For this review, take the finished solid that the model builds, in its own axes (mm). A direction names the side the tool comes from. Give positions to 0.01 mm unless a question says otherwise; leave off trailing zeros. Loops run counter-clockwise (first coordinate to the right, second up) from the corner with the lowest first, then second, coordinate; pieces in that order, holes last. Notation, with made-up numbers: (67.5, 31) - (83.5, 31) arc R15 cw to (83.5, 38) - close; hole circle Ø3 at (14, -9). An arc over 180 degrees is marked (long way). Put each result on its own line as item: value.
from build123d import *

# Parameters (mm, degrees)
BASPROSKE_W         = 44.5
BASPROSKE_H         = 30
TOOTHCUT_DEPTH      = 62.483737687
TEETHCUTS_COUNT     = 22
TEETHCUTS_ANGLE     = 343.636363636
HUBNEAONESKE_R      = 21
HUBNEARONE_DEPTH    = 5.5000508
BORSKE_R            = 12
BORE_DEPTH          = 50.0000508
CUT_EXTRUDE1_START  = -15.41
SKETCH1_R           = 30
CUT_EXTRUDE1_DEPTH  = 15.41
BOSS_EXTRUDE1_START = -3.95
SKETCH2_R           = 12
BOSS_EXTRUDE1_DEPTH = 3.95
SKETCH3_R           = 1.26
CUT_EXTRUDE2_DEPTH  = 55.622234789
SKETCH4_R           = 17.7
CUT_EXTRUDE3_DEPTH  = 30.64


with BuildPart() as part:
    # BasProSke → Base-Revolve (revolve)
    with BuildSketch(Plane(origin=(0, 0, 0), x_dir=(1, 0, 0), z_dir=(0, 1, 0)), mode=Mode.PRIVATE) as base_revolve_sk:
        with Locations((22.25, 15)):
            Rectangle(BASPROSKE_W, BASPROSKE_H)
    revolve(base_revolve_sk.sketch.rotate(Axis((-10, 0, 0), (1, 0, 0)), 180), axis=Axis((-10, 0, 0), (1, 0, 0)))

    # TooCutSke → ToothCut (cut, through all)
    with BuildSketch(Plane(origin=(0, 0, 0), x_dir=(0, 0, -1), z_dir=(1, 0, 0))):
        with BuildLine():
            ThreePointArc((1.215293185, 24.343683749), (0, 24.374), (-1.215293185, 24.343683749))
            ThreePointArc((-1.215293185, 24.343683749), (-2.034367134, 27.241050063), (-3.608361155, 29.807790507))
            ThreePointArc((-3.608361155, 29.807790507), (0, 30.0254), (3.608361155, 29.807790507))
            ThreePointArc((3.608361155, 29.807790507), (2.034367134, 27.241050063), (1.215293185, 24.343683749))
        make_face()
    toothcut = extrude(amount=TOOTHCUT_DEPTH, mode=Mode.SUBTRACT)

    # TeethCuts: ToothCut ×22 about axis
    teethcuts_axis = Axis((-10, 0, 0), (1, 0, 0))
    for i in range(1, TEETHCUTS_COUNT):
        add(toothcut.rotate(teethcuts_axis, i * TEETHCUTS_ANGLE / (TEETHCUTS_COUNT - 1)), mode=Mode.SUBTRACT)

    # HubNeaOneSke → HubNearOne (add)
    with BuildSketch(Plane.ZY):
        with Locations(Location((0, 0, 0), (0, 0, 180))):
            Circle(HUBNEAONESKE_R)
    extrude(amount=HUBNEARONE_DEPTH)

    # BorSke → Bore (cut, symmetric)
    with BuildSketch(Plane(origin=(0, 0, 0), x_dir=(0, 0, -1), z_dir=(1, 0, 0))):
        with Locations(Location((0, 0, 0), (0, 0, 180))):
            Circle(BORSKE_R)
    extrude(amount=BORE_DEPTH, both=True, mode=Mode.SUBTRACT)

    # Sketch1 → Cut-Extrude1 (cut)
    with BuildSketch(Plane.ZY.offset(5.5000508).offset(CUT_EXTRUDE1_START)):
        Circle(SKETCH1_R)
    extrude(amount=CUT_EXTRUDE1_DEPTH, mode=Mode.SUBTRACT)

    # Sketch2 → Boss-Extrude1 (add)
    with BuildSketch(Plane.ZY.offset(-9.9099492).offset(BOSS_EXTRUDE1_START)):
        Circle(SKETCH2_R)
    extrude(amount=BOSS_EXTRUDE1_DEPTH)

    # Sketch3 → Cut-Extrude2 (cut, through all)
    with BuildSketch(Plane.ZY.offset(-9.9099492)):
        with Locations((0, 8)):
            Circle(SKETCH3_R)
        with Locations((6.92820323, 4)):
            Circle(SKETCH3_R)
        with Locations((6.92820323, -4)):
            Circle(SKETCH3_R)
        with Locations((0, -8)):
            Circle(SKETCH3_R)
        with Locations((-6.92820323, -4)):
            Circle(SKETCH3_R)
        with Locations((-6.92820323, 4)):
            Circle(SKETCH3_R)
    extrude(amount=-CUT_EXTRUDE2_DEPTH, mode=Mode.SUBTRACT)

    # Sketch4 → Cut-Extrude3 (cut)
    with BuildSketch(Plane(origin=(44.5, 0, 0), x_dir=(0, 0, -1), z_dir=(1, 0, 0))):
        Circle(SKETCH4_R)
    extrude(amount=-CUT_EXTRUDE3_DEPTH, mode=Mode.SUBTRACT)


solid = part.part
1) For faces 5 (the face through (26.963, -13.187, -23.952)), 6 (the face through (26.96, -26.74, -5.72)), 7 (the face through (26.963, -21.785, -16.392)), list the 3-axis set-ups (+Z, -Z, +X, -X, +Y, -Y) from which the entire face can be reached by the end or side of a thin tool; tool diameter is ignored.
Geometry check:
face 5: -Z, +X, -X
face 6: +X, -X
face 7: +X, -X, -Y
2) Take a section at A-A on z = 0. State how many separate pieces and enclosed holes the cut face has, and give its area (3 significant figures).
Geometry check:
separate pieces: 3
enclosed holes: 0
area: 582 mm²
3) Insertion check: pin 1 Ø1 at (x, z) = (21.5, -24) entering from +Y; pin 2 Ø1.5 at (y, z) = (-8, 0) entering from +X (3 decimals); pin 3 Ø3 at (x, y) = (39.5, -2) entering from +Z; pin 4 Ø1.5 at (y, z) = (5.5, -5.5) entering from +X. Each pin has a flat end and moves straight along its axis. Give the tip position at first contact, or say it passes through.
Geometry check:
pin 1: stops at y = 16.78
pin 2: passes through
pin 3: stops at z = 30
pin 4: stops at x = 13.86
4) Wall thickness on line 1 (Y direction, x = 35, z = -26); line 2 (Y direction, x = 16, z = -22.5); line 3 (Y direction, x = 22, z = 9): over which ranges is each line inside the solid? List them lowest first.
Geometry check:
line 1: y = -9.47 to -5.5, -2.13 to 2.13, 5.5 to 9.47
line 2: y = -16.46 to -11.83, -9.37 to 9.37, 11.83 to 16.46
line 3: y = -24.74 to -15.24, 15.24 to 24.74
5) Take a section at B-B on y = 13.5. State the section outline as (x, z) points.
Geometry check:
outline: (9.91, -24.22) - (44.5, -24.22) - (44.5, -11.45) - (13.86, -11.45) - (13.86, 11.45) - (44.5, 11.45) - (44.5, 24.22) - (9.91, 24.22) - close
6) Draft analysis for pull direction Y (two halves, no side actions). For faces 1 (the face through (26.963, -13.124, 23.896)), 2 (the face through (9.91, 0, 0)), 3 (the face through (26.96, -27.19, -2.01)), 4 (the face through (26.96, 27.19, 2.01)), state which applies: pulls with the +Y half, pulls with the -Y half, needs draft (parallel to the pull), parting line crosses it, or undercut.
Geometry check:
face 1: undercut
face 2: needs draft
face 3: pulls with the -Y half
face 4: pulls with the +Y half
